Autodesk Inventor part; units mm, degrees
ref_plane "Work Plane1" through (0, 18.542, 0) normal (0, 1, 0) x (1, 0, 0)
ref_plane "YZ Plane" through (0, 0, 0) normal (1, 0, 0) x (0, 1, 0)
ref_plane "XZ Plane" through (0, 0, 0) normal (0, 1, 0) x (-1, 0, 0)
sketch "Sketch1" plane through (0, 0, 0) normal (0, 1, 0) x (-1, 0, 0)
  line L0 (1.27, 0) -> (11.43, 0)
  line L1 (12.7, -1.27) -> (12.7, -21.59)
  line L2 (11.43, -22.86) -> (1.27, -22.86)
  line L3 (0, -21.59) -> (0, -1.27)
  arc A0 (12.7, -1.27) -> (11.43, 0) centre (11.43, -1.27) ccw
  arc A1 (1.27, 0) -> (0, -1.27) centre (1.27, -1.27) ccw
  arc A2 (0, -21.59) -> (1.27, -22.86) centre (1.27, -21.59) ccw
  arc A3 (11.43, -22.86) -> (12.7, -21.59) centre (11.43, -21.59) ccw
  point P0 (0, 0)
  point P1 (12.7, -22.86)
  point P2 (12.7, 0)
  point P3 (0, -22.86)
  dimension "d0" = 12.7
  dimension "d1" = 22.86
  dimension "d2" = 1.27
extrude "Extrusion1" add sketch "Sketch1" along normal blind 22.86
sketch "Sketch2" plane through (0, 22.86, 0) normal (0, 1, 0) x (1, 0, 0)
  line L0 (-12.7, 21.59) -> (-12.7, 1.27)
  line L1 (-11.43, 0) -> (-1.27, 0)
  line L2 (0, 1.27) -> (0, 21.59)
  circle A0 centre (-6.35, 6.35) radius 6.35
  point P0 (0, 0)
extrude "Extrusion2" add sketch "Sketch2" along normal blind 5.08
ref_plane "Work Plane1" through (0, 18.542, 0) normal (0, 1, 0) x (1, 0, 0)
sketch "Sketch5" plane through (0, 18.542, 0) normal (0, 1, 0) x (1, 0, 0)
  line L0 (-12.7, 27.432) -> (0, 27.432)
  line L1 (-12.7, 21.59) -> (-12.7, 1.27)
  line L2 (0, 1.27) -> (0, 21.59)
  circle A0 centre (-6.35, 24.13) radius 1.016
  line L3 (0, 11.43) -> (-12.7, 11.43) construction
  line L4 (-12.7, -4.572) -> (0, -4.572)
  circle A1 centre (-6.35, -1.27) radius 1.016
  line L5 (-12.7, -4.572) -> (-12.7, 27.432)
  line L6 (0, 27.432) -> (0, -4.572)
  point P0 (0, 0)
  dimension "d13" = 16.002
  dimension "d14" = 2.032
  dimension "d15" = 25.4
extrude "Extrusion4" add sketch "Sketch5" against normal blind 2.54
sketch "Sketch6" plane through (-11.43, 0, 0) normal (0, 0, 1) x (1, 0, 0)
  line L0 (3.429, 5.334) -> (6.731, 5.334)
  line L1 (6.731, 5.334) -> (6.731, 4.318)
  line L2 (6.731, 4.318) -> (3.429, 4.318)
  line L3 (3.429, 4.318) -> (3.429, 5.334)
  line L4 (0, 0) -> (10.16, 0)
  point P0 (11.43, 0)
  point P1 (5.08, 0)
  point P2 (5.08, 4.318)
  dimension "d18" = 3.302
  dimension "d19" = 1.016
  dimension "d20" = 4.318
extrude "Extrusion5" add sketch "Sketch6" along normal blind 2.54
sketch "Sketch7" plane through (-6.35, 27.94, -6.35) normal (0, 1, 0) x (1, 0, 0)
  circle A0 centre (0, 0) radius 2.5
  point P0 (6.35, -6.35)
  dimension "d23" = 5
extrude "Extrusion6" add sketch "Sketch7" along normal blind 3
properties part number "servo (2)"
Work out the finished part from the listing and answer in its coordinate system (mm). A direction names the side the tool comes from. Coordinates: 2 decimals unless noted, no trailing zeros. Loops run counter-clockwise (first coordinate to the right, second up) from the corner with the lowest first, then second, coordinate; pieces in that order, holes last. Notation, with made-up numbers: (19, 17.5) -> (44, 17.5) arc R19 cw to (44, 45.5) -> close; hole circle Ø3 at (41, 45.5). An arc over 180 degrees is marked (long way). Answer as CSV lines item,"result".
Q1. The part is cut by section D-D on x = -11. Write down the section's boundary in (y, z), and give its area (3 significant figures).
Findings:
outline,"(0, -22.86) -> (16, -22.86) -> (16, -27.43) -> (18.54, -27.43) -> (18.54, -22.86) -> (22.86, -22.86) -> (22.86, -10.67) -> (27.94, -10.67) -> (27.94, -2.03) -> (22.86, -2.03) -> (22.86, 0) -> (18.54, 0) -> (18.54, 4.57) -> (16, 4.57) -> (16, 0) -> (0, 0) -> close"
area,"590 mm²"
Q2. Each of these flat-tipped pins is pushed along its axis until it touches: pin 1 (4.5 mm diameter, centred on x = -4.5, z = 1.5, fed in from +Y); pin 2 (1.5 mm diameter, centred on x = -4, y = 24, fed in from +Z); pin 3 (2 mm diameter, centred on x = -7.5, y = 11.5, fed in from -Z). Where does it stop, or does it pass through?
Findings:
pin 1,"stops at y = 27.94"
pin 2,"stops at z = -0.2"
pin 3,"stops at z = -22.86"
Q3. The part is cut by section B-B on y = 11.5. Write down the section's boundary in (x, z), and give its area (3 significant figures).
Findings:
outline,"(-12.7, -21.59) arc R1.27 ccw to (-11.43, -22.86) -> (-1.27, -22.86) arc R1.27 ccw to (0, -21.59) -> (0, -1.27) arc R1.27 ccw to (-1.27, 0) -> (-11.43, 0) arc R1.27 ccw to (-12.7, -1.27) -> close"
area,"289 mm²"
Q4. The part is cut by section A-A on z = -24.13. Write down the section's boundary in (x, y).
Findings:
outline,"(-12.7, 16) -> (-7.37, 16) -> (-7.37, 18.54) -> (-12.7, 18.54) -> close; (-5.33, 16) -> (0, 16) -> (0, 18.54) -> (-5.33, 18.54) -> close"
Q5. Find the intervals of material crossed by probe 1 along Z at (x, y) = (-6.35, 16.75); probe 2 along Z at (x, y) = (-5.5, 16.5); probe 3 along X at (y, z) = (17.85, -24.13), in increasing order.
Findings:
probe 1,"z = -27.43 to -25.15, -23.11 to 0.25, 2.29 to 4.57"
probe 2,"z = -27.43 to -24.69, -23.57 to 0.71, 1.83 to 4.57"
probe 3,"x = -12.7 to -7.37, -5.33 to 0"
Q6. The part is cut by section C-C on z = 1.27. Write down the section's boundary in (x, y).
Findings:
outline,"(-12.7, 16) -> (-7.37, 16) -> (-7.37, 18.54) -> (-12.7, 18.54) -> close; (-8, 4.32) -> (-4.7, 4.32) -> (-4.7, 5.33) -> (-8, 5.33) -> close; (-5.33, 16) -> (0, 16) -> (0, 18.54) -> (-5.33, 18.54) -> close"
Q7. A tool of negligible diameter and unlimited length cuts with its end or side. For faces 1 (the face through (-12.338, 20.671, -22.478)), 2 (the face through (-0.484, 25.364, -8.782)), 3 (the face through (-6, 4.318, 1)), 4 (the face through (-11.2, 22.86, -1.5)), from which of +Z, -Z, +X, -X, +Y, -Y can it reach the whole face along a straight path? Write none if from no direction.
Findings:
face 1,"-Z, -X, +Y"
face 2,"+Y"
face 3,"+Z, +X, -X, -Y"
face 4,"+Z, -X, +Y"
Q8. For a pull along Y with two mould halves and no side action, classify faces 5 (the face through (-6, 8, 0)), 6 (the face through (-6, 18.542, -26)), 7 (the face through (-6, 21, 0)) as +Y half, -Y half, draft (parallel to the pull), parting line (faces both ways), or undercut.
Findings:
face 5,"undercut"
face 6,"+Y half"
face 7,"draft"
